```python
from build123d import *

# Parameters (mm, degrees)
F0_R     = 1.5875
F1_DEPTH = 25.4


with BuildPart() as f1:
    # F0 (on Front) → F1 (new body)
    with BuildSketch(Plane.XZ):
        with BuildLine():
            Line((3.175, 0), (9.525, 0))
            ThreePointArc((9.525, 0), (6.7351920908, 6.7351920908), (0, 9.525))
            Line((0, 9.525), (0, 3.175))
            ThreePointArc((0, 3.175), (2.2450640303, 2.2450640303), (3.175, 0))
        make_face()
        with BuildLine():
            Line((36.5125, 0), (9.525, 0))
            ThreePointArc((9.525, 0), (6.9705567315, -6.4912990883), (0.6773435479, -9.500885786))
            Line((0.6773435479, -9.500885786), (44.7324052746, -7.9324746146))
            ThreePointArc((44.7324052746, -7.9324746146), (38.9380895153, -5.7116327839), (36.5125, 0))
        make_face()
        with BuildLine():
            ThreePointArc((0.6773435479, -9.500885786), (6.9705567315, -6.4912990883), (9.525, 0))
            Line((9.525, 0), (3.175, 0))
            ThreePointArc((3.175, 0), (-2.2450640303, -2.2450640303), (0, 3.175))
            Line((0, 3.175), (0, 9.525))
            ThreePointArc((0, 9.525), (-9.525, 0), (0, -9.525))
            Line((0, -9.525), (0.6773435479, -9.500885786))
        make_face()
        with BuildLine():
            ThreePointArc((0, 9.525), (6.7351920908, 6.7351920908), (9.525, 0))
            Line((9.525, 0), (36.5125, 0))
            ThreePointArc((36.5125, 0), (38.9380895153, 5.7116327839), (44.7324052746, 7.9324746146))
            Line((44.7324052746, 7.9324746146), (18.9341027877, 8.850924033))
            ThreePointArc((18.9341027877, 8.850924033), (13.2249738114, 11.5709798305), (11.3072231466, 17.5971800924))
            Line((11.3072231466, 17.5971800924), (15.7942028036, 61.9003804205))
            ThreePointArc((15.7942028036, 61.9003804205), (10.644756084, 51.722700101), (0, 47.625))
            Line((0, 47.625), (0, 9.525))
        make_face()
        with BuildLine():
            ThreePointArc((0, -9.525), (0.3388863295, -9.5189695375), (0.6773435479, -9.500885786))
            Line((0.6773435479, -9.500885786), (0, -9.525))
        make_face()
        with BuildLine():
            ThreePointArc((44.7324052746, 7.9324746146), (38.9380895153, 5.7116327839), (36.5125, 0))
            ThreePointArc((36.5125, 0), (38.9380895153, -5.7116327839), (44.7324052746, -7.9324746146))
            ThreePointArc((44.7324052746, -7.9324746146), (50.1616327839, -5.5119104847), (52.3875, 0))
            ThreePointArc((52.3875, 0), (50.1616327839, 5.5119104847), (44.7324052746, 7.9324746146))
        make_face()
        with BuildLine():
            ThreePointArc((47.625, 0), (44.45, -3.175), (41.275, 0))
            ThreePointArc((41.275, 0), (44.45, 3.175), (47.625, 0))
        make_face(mode=Mode.SUBTRACT)
        with BuildLine():
            Line((0, 60.325), (0, 47.625))
            ThreePointArc((0, 47.625), (10.644756084, 51.722700101), (15.7942028036, 61.9003804205))
            Line((15.7942028036, 61.9003804205), (15.7942028036, 65.0996195795))
            Line((15.7942028036, 65.0996195795), (15.6978424192, 65.8650303134))
            ThreePointArc((15.6978424192, 65.8650303134), (10.3554519161, 75.5324661069), (0, 79.375))
            Line((0, 79.375), (0, 66.675))
            ThreePointArc((0, 66.675), (2.2450640303, 65.7450640303), (3.175, 63.5))
            ThreePointArc((3.175, 63.5), (2.2450640303, 61.2549359697), (0, 60.325))
        make_face()
        with BuildLine():
            ThreePointArc((-15.7501779217, 61.5131632086), (-10.4993950049, 51.5929294311), (0, 47.625))
            Line((0, 47.625), (0, 60.325))
            ThreePointArc((0, 60.325), (-3.175, 63.5), (0, 66.675))
            Line((0, 66.675), (0, 79.375))
            ThreePointArc((0, 79.375), (-10.4993950049, 75.4070705689), (-15.7501779217, 65.4868367914))
            Line((-15.7501779217, 65.4868367914), (-15.7501779217, 61.5131632086))
        make_face()
        with BuildLine():
            ThreePointArc((-15.7501779217, 65.4868367914), (-15.875, 63.5), (-15.7501779217, 61.5131632086))
            Line((-15.7501779217, 61.5131632086), (-15.7501779217, 65.4868367914))
        make_face()
        with BuildLine():
            Line((15.7942028036, 65.0996195795), (15.7942028036, 61.9003804205))
            ThreePointArc((15.7942028036, 61.9003804205), (15.8547878338, 62.6991705884), (15.875, 63.5))
            ThreePointArc((15.875, 63.5), (15.8547878338, 64.3008294116), (15.7942028036, 65.0996195795))
        make_face()
        with BuildLine():
            Line((-9.4907647262, 115.1068518528), (-15.7501779217, 65.4868367914))
            ThreePointArc((-15.7501779217, 65.4868367914), (-10.4993950049, 75.4070705689), (0, 79.375))
            Line((0, 79.375), (0, 104.775))
            ThreePointArc((0, 104.775), (-7.0146592539, 107.8563845125), (-9.4907647262, 115.1068518528))
        make_face()
        with Locations((-7.1771577932, 100.0252)):
            Circle(F0_R, mode=Mode.SUBTRACT)
        with BuildLine():
            Line((15.6978424192, 65.8650303134), (15.7942028036, 65.0996195795))
            ThreePointArc((15.7942028036, 65.0996195795), (15.7506727309, 65.4829103672), (15.6978424192, 65.8650303134))
        make_face()
        with BuildLine():
            Line((0, 104.775), (0, 79.375))
            ThreePointArc((0, 79.375), (10.3554519161, 75.5324661069), (15.6978424192, 65.8650303134))
            Line((15.6978424192, 65.8650303134), (9.4504036385, 115.4897462203))
            ThreePointArc((9.4504036385, 115.4897462203), (9.5063326172, 114.8960412498), (9.525, 114.3))
            ThreePointArc((9.525, 114.3), (6.7351920908, 107.5648079092), (0, 104.775))
        make_face()
        with BuildLine():
            Line((-9.393817197, 115.8753804205), (-9.4907647262, 115.1068518528))
            ThreePointArc((-9.4907647262, 115.1068518528), (-7.0146592539, 107.8563845125), (0, 104.775))
            ThreePointArc((0, 104.775), (6.7351920908, 107.5648079092), (9.525, 114.3))
            ThreePointArc((9.525, 114.3), (9.5063326172, 114.8960412498), (9.4504036385, 115.4897462203))
            ThreePointArc((9.4504036385, 115.4897462203), (0.1948818628, 123.8230061461), (-9.393817197, 115.8753804205))
        make_face()
        with BuildLine():
            ThreePointArc((3.175, 114.3), (2.2450640303, 112.0549359697), (0, 111.125))
            ThreePointArc((0, 111.125), (-2.2450640303, 116.5450640303), (3.175, 114.3))
        make_face(mode=Mode.SUBTRACT)
        with BuildLine():
            ThreePointArc((-9.393817197, 115.8753804205), (-9.450106753, 115.4921020748), (-9.4907647262, 115.1068518528))
            Line((-9.4907647262, 115.1068518528), (-9.393817197, 115.8753804205))
        make_face()
    extrude(amount=F1_DEPTH)


solid = f1.part
```
For this review, take the finished solid that the model builds, in its own axes (mm). A direction names the side the tool comes from. Coordinates: 2 decimals unless noted, no trailing zeros. Write each loop counter-clockwise with the first axis right and the second up, starting at its lowest first coordinate (ties: lowest second). Pieces come first, ordered by that corner, then holes.
(1) Add section B-B on z = 113. Give the boundary of the cut face in (x, y).
(2) Wall thickness on probe 1 along Z at (x, y) = (44.45, -8.5) (3 decimals); probe 2 along X at (y, z) = (-1.25, 2); probe 3 along Z at (x, y) = (43.5, -12): over which ranges is each line inside the solid? List them lowest first.
(3) Add section D-D on z = 69.5. Give the boundary of the cut face in (x, y).
(4) Add section A-A on x = 13.5. Give the boundary of the cut face in (y, z), then the cut area to 3 significant figures.
(5) Add section C-C on y = -21.75. Count the separate pieces of the cut face and the enclosed holes in it, then the cut area to 3 significant figures.
(6) Tool access review of faces 4 (the face through (13.52, -12.52, 39.44)), 5 (the face through (0, -13, 29)), 6 (the face through (10, 0, 58)): name each direction out of +Z, -Z, +X, -X, +Y, -Y from which nothing blocks a thin tool from reaching the whole face with its end or side.
(7) The part is to be moulded in two halves that separate along Z. For faces 1 (the face through (-12.577, -12.522, 90.644)), 2 (the face through (10, -25.4, 58)), 3 (the face through (13.29, -12.52, 11.5)), say which applies: +Z half, -Z half, draft (parallel to the pull), parting line (faces both ways), or undercut.
(8) For pin 1 Ø12.5 at (y, z) = (-15, 23.5) entering from -X; pin 2 Ø2 at (y, z) = (-3, 51.5) entering from +X; pin 3 Ø2 at (x, y) = (21, -14) entering from -Z, all flat-tipped, find the tip position at first contact; note any pin that passes through.
Answer sheet:
1. outline: (-9.76, -25.4) - (-2.9, -25.4) - (-2.9, 0) - (-9.76, 0) - close; (2.9, -25.4) - (9.76, -25.4) - (9.76, 0) - (2.9, 0) - close
2. probe 1: z = -7.943 to -3.175, 3.175 to 7.943
2. probe 2: x = -9.31 to -2.47, 2.47 to 41.98, 46.92 to 52.13
2. probe 3: z = -7.98 to -3.03, 3.03 to 7.98
3. outline: (-15.24, -25.4) - (15.24, -25.4) - (15.24, 0) - (-15.24, 0) - close
4. outline: (-25.4, -9.04) - (0, -9.04) - (0, 11.27) - (-25.4, 11.27) - close; (-25.4, 39.25) - (0, 39.25) - (0, 83.32) - (-25.4, 83.32) - close
4. area: 1,640 mm2
5. separate pieces: 1
5. enclosed holes: 5
5. area: 3,260 mm2
6. face 4: +X, +Y, -Y
6. face 5: -X, +Y, -Y
6. face 6: +Z, -Z, +X, -X, +Y
7. face 1: +Z half
7. face 2: draft
7. face 3: undercut
8. pin 1: stops at x = 0
8. pin 2: stops at x = 14.84
8. pin 3: stops at z = -8.81
